```python
from build123d import *

# Parameters (mm, degrees)
SKETCH1_R           = 1.8
SKETCH1_R_2         = 2.3
BOSS_EXTRUDE1_DEPTH = 3
BOSS_EXTRUDE2_START = 3
SKETCH1_4_R         = 1.25
BOSS_EXTRUDE2_DEPTH = 2
BOSS_EXTRUDE3_START = 5
BOSS_EXTRUDE3_DEPTH = 2
FILLET1_R           = 2
FILLET2_R           = 2


with BuildPart() as part:
    # Sketch1 → Boss-Extrude1 (new body)
    with BuildSketch(Plane.XY):
        with BuildLine():
            Line((-44.4, 14.4), (-44.4, -14.4))
            Line((-44.4, -14.4), (-29.4, -14.4))
            Line((-29.4, -14.4), (-29.4, 10.441638902))
            ThreePointArc((-29.4, 10.441638902), (-25.775066243, 15.752493555), (-31.408334135, 18.852753985))
            Line((-31.408334135, 18.852753985), (-44.4, 14.4))
        make_face()
        with Locations((-30, 14.7437)):
            Circle(SKETCH1_R, mode=Mode.SUBTRACT)
        with Locations((-38, 8)):
            Circle(SKETCH1_R_2, mode=Mode.SUBTRACT)
        with Locations((-38, -8)):
            Circle(SKETCH1_R_2, mode=Mode.SUBTRACT)
    extrude(amount=BOSS_EXTRUDE1_DEPTH)

    # Sketch1<4> → Boss-Extrude2 (add)
    with BuildSketch(Plane.XY.offset(BOSS_EXTRUDE2_START)):
        with BuildLine():
            Line((-29.4, -14.4), (-29.4, 10.441638902))
            ThreePointArc((-29.4, 10.441638902), (-32.719472632, 11.356636627), (-34.330080831, 14.4))
            Line((-34.330080831, 14.4), (-44.4, 14.4))
            Line((-44.4, 14.4), (-44.4, -14.4))
            Line((-44.4, -14.4), (-29.4, -14.4))
        make_face()
        with Locations((-38, -8)):
            Circle(SKETCH1_4_R, mode=Mode.SUBTRACT)
        with Locations((-38, 8)):
            Circle(SKETCH1_4_R, mode=Mode.SUBTRACT)
    extrude(amount=BOSS_EXTRUDE2_DEPTH)

    # Sketch1<5> → Boss-Extrude3 (add)
    with BuildSketch(Plane.XY.offset(BOSS_EXTRUDE3_START)):
        with BuildLine():
            Line((-29.4, -14.4), (-29.4, -10.4))
            Line((-29.4, -10.4), (-40.4, -10.4))
            Line((-40.4, -10.4), (-40.4, 10.4))
            Line((-40.4, 10.4), (-30, 10.4))
            ThreePointArc((-30, 10.4), (-32.947439567, 11.553037108), (-34.330080831, 14.4))
            Line((-34.330080831, 14.4), (-44.4, 14.4))
            Line((-44.4, 14.4), (-44.4, -14.4))
            Line((-44.4, -14.4), (-29.4, -14.4))
        make_face()
    extrude(amount=BOSS_EXTRUDE3_DEPTH)

    # Fillet1
    fillet1_edges = [part.edges().sort_by_distance(p)[0] for p in [
        (-29.4, -14.4, 3.5),
        (-44.4, -14.4, 3.5),
        (-44.4, 14.4, 5),
    ]]
    fillet(fillet1_edges, radius=FILLET1_R)

    # Fillet2
    fillet2_edges = [part.edges().sort_by_distance(p)[0] for p in [
        (-44.4, 14.4, 1.5),
    ]]
    fillet(fillet2_edges, radius=FILLET2_R)


solid = part.part
```
Here's how the part is built. I have some questions about the finished solid (model axes, mm). A direction names the side the tool comes from. Give positions to 0.01 mm unless a question says otherwise; leave off trailing zeros. Loops run counter-clockwise (first coordinate to the right, second up) from the corner with the lowest first, then second, coordinate; pieces in that order, holes last. Notation, with made-up numbers: M -6,30 L 49,30 A15 cw 49,34 Z; hole C 62.5,42 d9. An arc over 180 degrees is marked long. Return JSON: item names as keys, results as strings.
Item 1: Imagine slicing it at A-A on y = -8. List the corners of the cut face in (x, z) for me.
A:
{"outline": "M -44.4,0 L -40.3,0 L -40.3,3 L -39.25,3 L -39.25,5 L -40.4,5 L -40.4,7 L -44.4,7 Z; M -36.75,3 L -35.7,3 L -35.7,0 L -29.4,0 L -29.4,5 L -36.75,5 Z"}
Item 2: On a 3-axis mill with a long thin cutter (end or side, diameter ignored), from which of +Z, -Z, +X, -X, +Y, -Y can I reach the whole of each face in a straight line? I mean faces 1 (the cylindrical face through (-43.8, 13.83, 4.97)), 2 (the flat face through (-35, 10.4, 6)), 3 (the cylindrical face through (-40.298, -7.899, 1.479)), 4 (the flat face through (-38, 14.4, 5)), 5 (the flat face through (-29.4, -1, 3)). Say none if no direction works.
A:
{"face 1": "+Z, -X, +Y", "face 2": "+Z, +X", "face 3": "-Z", "face 4": "+Z, +X, -X, +Y", "face 5": "+Z, -Z, +X, -Y"}
Item 3: Imagine slicing it at C-C on z = 5.5. List the corners of the cut face in (x, y) for me.
A:
{"outline": "M -44.4,-12.4 A2 ccw -42.4,-14.4 L -31.4,-14.4 A2 ccw -29.4,-12.4 L -29.4,-10.4 L -40.4,-10.4 L -40.4,10.4 L -30,10.4 A4.34 cw -34.33,14.4 L -42.4,14.4 A2 ccw -44.4,12.4 Z"}
Item 4: I'm going to push flat-ended pins straight in: pin 1 Ø3 at (x, y) = (-38, 8) entering from +Z; pin 2 Ø1 at (x, z) = (-36.5, 6) entering from +Y; pin 3 Ø0.6 at (y, z) = (4.5, 6) entering from +X; pin 4 Ø2 at (x, y) = (-30, 14.74) entering from +Z. Where does each tip first touch, or does it pass through?
A:
{"pin 1": "stops at z = 5", "pin 2": "stops at y = 14.4", "pin 3": "stops at x = -40.4", "pin 4": "passes through"}
Item 5: Thinking about a two-plate mould opening in Y: for faces 6 (the flat face through (-33, 15, 3)), 7 (the flat face through (-37, -9, 3)), 8 (the cylindrical face through (-25.75, 15.65, 1.48)), which applies, released by +Y, released by -Y, zero draft, split by the parting line, or undercut?
A:
{"face 6": "zero draft", "face 7": "undercut", "face 8": "split by the parting line"}
Item 6: Imagine slicing it at B-B on x = -38. List the corners of the cut face in (y, z) for me.
A:
{"outline": "M -14.4,0 L -10.3,0 L -10.3,3 L -9.25,3 L -9.25,5 L -10.4,5 L -10.4,7 L -14.4,7 Z; M -6.75,3 L -5.7,3 L -5.7,0 L 5.7,0 L 5.7,3 L 6.75,3 L 6.75,5 L -6.75,5 Z; M 9.25,3 L 10.3,3 L 10.3,0 L 16.59,0 L 16.59,3 L 14.4,3 L 14.4,7 L 10.4,7 L 10.4,5 L 9.25,5 Z"}
Item 7: Please list where these lines run through material, in increasing order: line 1 (Y direction, x = -38, z = 4.05); line 2 (Y direction, x = -35.5, z = 6); line 3 (Y direction, x = -38, z = 1).
A:
{"line 1": "y = -14.4 to -9.25, -6.75 to 6.75, 9.25 to 14.4", "line 2": "y = -14.4 to -10.4, 10.4 to 14.4", "line 3": "y = -14.4 to -10.3, -5.7 to 5.7, 10.3 to 16.59"}
Item 8: Imagine slicing it at D-D on z = 2.25. List the corners of the cut face in (x, y) for me, then the cut area to 3 significant figures.
A:
{"outline": "M -44.4,-12.4 A2 ccw -42.4,-14.4 L -31.4,-14.4 A2 ccw -29.4,-12.4 L -29.4,10.44 A4.34 ccw long -31.41,18.85 L -43.05,14.86 A2 ccw -44.4,12.97 Z; hole C -38,-8 d4.6; hole C -38,8 d4.6; hole C -30,14.74 d3.6", "area": "449 mm^2"}
